Geometry: final body of the model. Coordinates: model frame, mm. A direction names the side the tool comes from. Give positions to 0.01 mm unless a question says otherwise; leave off trailing zeros. Write each loop counter-clockwise with the first axis right and the second up, starting at its lowest first coordinate (ties: lowest second). Pieces come first, ordered by that corner, then holes.
from build123d import *

# Parameters (mm, degrees)
F1_DEPTH = 5
F3_DEPTH = 5.401
F4_R     = 1.25
F5_DEPTH = 8.501
F6_R     = 0.9
F7_DEPTH = 7.7
F8_R     = 0.75
F9_DEPTH = 2.0010001


with BuildPart() as f1:
    # F0 (on Right) → F1 (new body)
    with BuildSketch(Plane.YZ):
        Polygon((9.7, 0), (0, 0), (0, -6), (5.1, -6), (5.1, -8.5), (9.7, -8.5), (9.7, -5.1), (13.7, -5.1), (13.7, -4.4), (9.9, -4.4), (9.9, -3.8), (13.7, -3.8), (13.7, -3.1), (9.7, -3.1), align=None)
    extrude(amount=F1_DEPTH)

    # F2 (on face) → F3 (cut, through all)
    with BuildSketch(Plane.XY.offset(-3.1)):
        with BuildLine():
            Line((1.1, 13.7), (1.1, 12.5))
            ThreePointArc((1.1, 12.5), (2.5, 11.1), (3.9, 12.5))
            Line((3.9, 12.5), (3.9, 13.7))
            Line((3.9, 13.7), (1.1, 13.7))
        make_face()
    extrude(amount=-F3_DEPTH, mode=Mode.SUBTRACT)

    # F4 (on face) → F5 (cut, through all)
    with BuildSketch(Plane.XY):
        with Locations((2.5, 6.7)):
            Circle(F4_R)
    extrude(amount=-F5_DEPTH, mode=Mode.SUBTRACT)

    # F6 (on face) → F7 (cut)
    with BuildSketch(Plane(origin=(0, 9.7, 0), x_dir=(-1, 0, 0), z_dir=(0, 1, 0))):
        with Locations((-2.5, -1.4)):
            Circle(F6_R)
    extrude(amount=-F7_DEPTH, mode=Mode.SUBTRACT)

    # F8 (on face) → F9 (cut, through all)
    with BuildSketch(Plane(origin=(0, 9.7, 0), x_dir=(-1, 0, 0), z_dir=(0, 1, 0))):
        with Locations((-2.5, -6.4)):
            Circle(F8_R)
    extrude(amount=-F9_DEPTH, mode=Mode.SUBTRACT)


solid = f1.part
Q1. Pull-direction query (X, two-part tool) for faces 1 (the flat face through (1.9, 9.7, -2.3)), 2 (the cylindrical face through (2.5, 11.1, -4.7)), 3 (the cylindrical face through (3.25, 8.71, -6.37)), 4 (the flat face through (0, 5, -3)); classes: released by +X, released by -X, zero draft, split by the parting line, or undercut.
Filled sheet:
face 1: zero draft
face 2: undercut
face 3: undercut
face 4: released by -X
Q2. Section C-C on z = -1.4. Output: boundary loops of the cut face in (x, y).
Filled sheet:
outline: (0, 0) - (5, 0) - (5, 9.7) - (3.4, 9.7) - (3.4, 7.57) arc R1.25 cw to (3.4, 5.83) - (3.4, 2) - (1.6, 2) - (1.6, 5.83) arc R1.25 cw to (1.6, 7.57) - (1.6, 9.7) - (0, 9.7) - close
Q3. Access query for faces 5 (the flat face through (2, 11, -4.4)), 6 (the flat face through (2, 3, -6)), 7 (the cylindrical face through (2.085, 3.943, -2.198)), 8 (the flat face through (2, 11, -5.1)). Directions: +Z, -Z, +X, -X, +Y, -Y. A direction counts if a zero-diameter tool reaches every point of the face in a straight line with its end or side. Return the directions, or none.
Filled sheet:
face 5: +X, -X, +Y
face 6: -Z, +X, -X, -Y
face 7: +Y
face 8: -Z, +X, -X, +Y
Q4. Section D-D on x = 4.4. Output: boundary loops of the cut face in (y, z).
Filled sheet:
outline: (0, -6) - (5.1, -6) - (5.1, -8.5) - (9.7, -8.5) - (9.7, -5.1) - (13.7, -5.1) - (13.7, -4.4) - (9.9, -4.4) - (9.9, -3.8) - (13.7, -3.8) - (13.7, -3.1) - (9.7, -3.1) - (9.7, 0) - (0, 0) - close
Q5. Section A-A on x = 2.5. Count the separate pieces of the cut face and the enclosed holes in it, plus the area to 3 significant figures.
Filled sheet:
separate pieces: 4
enclosed holes: 0
area: 38.5 mm2
Q6. Pin query (flat end, axial travel): P1, Ø3, axis at x = 1, y = 10, coming from the +Z side; P2, Ø1.4, axis at x = 2.5, z = -1, coming from the +Y side; P3, Ø2, axis at x = 2, y = 11.5, coming from the +Z side; P4, Ø0.8, axis at x = 2.5, z = -7.5, coming from the -Y side. Return the tip coordinate at first contact, or that it passes through.
Filled sheet:
P1: stops at z = 0
P2: stops at y = 9.7
P3: stops at z = -3.1
P4: stops at y = 5.1
Q7. Section B-B on y = 6.7. Output: boundary loops of the cut face in (x, z).
Filled sheet:
outline: (0, -8.5) - (1.25, -8.5) - (1.25, 0) - (0, 0) - close; (3.75, -8.5) - (5, -8.5) - (5, 0) - (3.75, 0) - close
Q8. Ray query, line 1 along Z through (x, y) = (2.5, 8.45); line 2 along Z through (x, y) = (4.65, 10.5); line 3 along X through (y, z) = (4.55, -1.4). Return the intervals inside material, ascending.
Filled sheet:
line 1: z = -8.5 to -7.15, -5.65 to -2.3, -0.5 to 0
line 2: z = -5.1 to -4.4, -3.8 to -3.1
line 3: x = 0 to 1.6, 3.4 to 5
